from build123d import *

# Parameters (mm, degrees)
SKETCH1_R      = 5.9
EXTRUDE1_DEPTH = 10
FILLET1_R      = 2.8
EXTRUDE2_DEPTH = 8
FILLET2_R      = 0.2
EXTRUDE3_DEPTH = 9.8


with BuildPart() as part:
    # Sketch1 → Extrude1 (new body)
    with BuildSketch(Plane.XY):
        Circle(SKETCH1_R)
    extrude(amount=-EXTRUDE1_DEPTH)

    # Fillet1
    fillet1_edges = [part.edges().sort_by_distance(p)[0] for p in [
        (-5.9, 0, 0),
    ]]
    fillet(fillet1_edges, radius=FILLET1_R)

    # Sketch2 → Extrude2 (cut)
    with BuildSketch(Plane.XY):
        Polygon((-0.905, 2.315), (0.905, 2.315), (0.905, 0.905), (2.09345294, 0.905), (2.09345294, -0.905), (0.905, -0.905), (0.905, -2.273521567), (-0.905, -2.273521567), (-0.905, -0.905), (-2.345549018, -0.905), (-2.345549018, 0.905), (-0.905, 0.905), align=None)
    extrude(amount=-EXTRUDE2_DEPTH, mode=Mode.SUBTRACT)

    # Fillet2
    fillet2_edges = [part.edges().sort_by_distance(p)[0] for p in [
        (-0.905, 1.61, 0),
        (-1.625274509, 0.905, 0),
        (-2.345549018, 0, 0),
        (-1.625274509, -0.905, 0),
        (-0.905, -1.589260784, 0),
        (0, -2.273521567, 0),
        (0.905, -1.589260784, 0),
        (1.49922647, -0.905, 0),
        (2.09345294, 0, 0),
        (1.49922647, 0.905, 0),
        (0.905, 1.61, 0),
        (0, 2.315, 0),
    ]]
    fillet(fillet2_edges, radius=FILLET2_R)

    # Sketch3 → Extrude3 (add)
    with BuildSketch(Plane(origin=(0, 0, -10), x_dir=(-1, 0, 0), z_dir=(0, 0, -1))):
        with BuildLine():
            Line((-3.196218134, 0.9), (-8.1, 0.9))
            ThreePointArc((-8.1, 0.9), (-9, 0), (-8.1, -0.9))
            Line((-8.1, -0.9), (-3.196218134, -0.9))
            Line((-3.196218134, -0.9), (-3.196218134, 0.9))
        make_face()
        with BuildLine():
            Line((0.9, 3.376286761), (-0.9, 3.376286761))
            Line((-0.9, 3.376286761), (-0.9, 8.65))
            ThreePointArc((-0.9, 8.65), (0, 9.55), (0.9, 8.65))
            Line((0.9, 8.65), (0.9, 3.376286761))
        make_face()
        with BuildLine():
            Line((3.340273036, 0.9), (8.1, 0.9))
            ThreePointArc((8.1, 0.9), (9, 0), (8.1, -0.9))
            Line((8.1, -0.9), (3.340273036, -0.9))
            Line((3.340273036, -0.9), (3.340273036, 0.9))
        make_face()
        with BuildLine():
            Line((-0.9, -3.358279899), (0.9, -3.358279899))
            Line((0.9, -3.358279899), (0.9, -8.65))
            ThreePointArc((0.9, -8.65), (0, -9.55), (-0.9, -8.65))
            Line((-0.9, -8.65), (-0.9, -3.358279899))
        make_face()
    extrude(amount=-EXTRUDE3_DEPTH)

    # Sketch6 → Cut-Revolve3 (revolve, cut)
    with BuildSketch(Plane(origin=(0, 0, 0), x_dir=(0, 0, -1), z_dir=(1, 0, 0))):
        Polygon((2.318539135, -9.900453163), (-0.04993414, -9.900453163), (0.123609111, -4.036856485), align=None)
    revolve(axis=Axis((0, 0, -10.502496707), (0, 0, 1)), mode=Mode.SUBTRACT)


solid = part.part
CAD build for the part. Positions are in the model's coordinates, mm. A direction names the side the tool comes from. Coordinates: 2 decimals unless noted, no trailing zeros. Loops run counter-clockwise (first coordinate to the right, second up) from the corner with the lowest first, then second, coordinate; pieces in that order, holes last. Notation, with made-up numbers: (47, 81) -> (101, 81) arc R23 cw to (101, 91) -> close; hole circle Ø1 at (-35.75, 54.5). An arc over 180 degrees is marked (long way). One line per item, written item: value.
1. Slice it at B-B on x = 0. Write the cut outline in (y, z) (3 decimals).
Answers:
outline: (-9.55, -10) -> (9.55, -10) -> (9.55, -2.187) -> (4.241, -0.2) -> (4.139, -0.2) arc R2.8 ccw to (3.1, 0) -> (2.515, 0) arc R0.2 ccw to (2.315, -0.2) -> (2.315, -8) -> (-2.274, -8) -> (-2.274, -0.2) arc R0.2 ccw to (-2.474, 0) -> (-3.1, 0) arc R2.8 ccw to (-4.139, -0.2) -> (-4.241, -0.2) -> (-9.55, -2.187) -> close
2. Slice it at C-C on z = -1. Write the cut outline in (x, y) (3 decimals).
Answers:
outline: (-6.314, -0.9) -> (-5.167, -0.9) arc R5.245 ccw to (-0.9, -5.167) -> (-0.9, -6.314) arc R6.378 ccw to (0.9, -6.314) -> (0.9, -5.167) arc R5.245 ccw to (5.167, -0.9) -> (6.314, -0.9) arc R6.378 ccw to (6.314, 0.9) -> (5.167, 0.9) arc R5.245 ccw to (0.9, 5.167) -> (0.9, 6.314) arc R6.378 ccw to (-0.9, 6.314) -> (-0.9, 5.167) arc R5.245 ccw to (-5.167, 0.9) -> (-6.314, 0.9) arc R6.378 ccw to start; hole (-2.346, -0.905) -> (-0.905, -0.905) -> (-0.905, -2.274) -> (0.905, -2.274) -> (0.905, -0.905) -> (2.093, -0.905) -> (2.093, 0.905) -> (0.905, 0.905) -> (0.905, 2.315) -> (-0.905, 2.315) -> (-0.905, 0.905) -> (-2.346, 0.905) -> close
3. Which spindle directions (+Z, -Z, +X, -X, +Y, -Y) get a long thin tool onto all of the face, cutting with end or side? Do faces 1 (the face through (-2.346, 0, -4)), 2 (the face through (-0.02, -9.55, -5.99)). Say none if no direction does.
Answers:
face 1: +Z
face 2: +Z, -Z, -Y
4. Drill centre lines: line 1 (Y direction, x = 0.5, z = -5) (3 decimals); line 2 (Y direction, x = -7.5, z = -4.75); line 3 (Z direction, x = 0.5, y = -1.75). Where is each one in solid material? Low to high. Write a range as [from, to].
Answers:
line 1: y = [-9.398, -2.274], [2.315, 9.398]
line 2: y = [-0.9, 0.9]
line 3: z = [-10, -8]
5. Flat gauge pins, fed straight in: P1, Ø1.2, axis at x = -2, z = -3.5, coming from the -Y side; P2, Ø5, axis at y = 7.5, z = -6, coming from the -X side; P3, Ø6, axis at x = -4, z = -7.5, coming from the +Y side. Where does each tip first touch, or does it go through?
Answers:
P1: stops at y = -5.73
P2: stops at x = -3.13
P3: stops at y = 5.81
6. Slice it at A-A on z = -6.5. Write the cut outline in (x, y) (3 decimals), and give its area (3 significant figures).
Answers:
outline: (-8.1, -0.9) -> (-5.831, -0.9) arc R5.9 ccw to (-0.9, -5.831) -> (-0.9, -8.65) arc R0.9 ccw to (0.9, -8.65) -> (0.9, -5.831) arc R5.9 ccw to (5.831, -0.9) -> (8.1, -0.9) arc R0.9 ccw to (8.1, 0.9) -> (5.831, 0.9) arc R5.9 ccw to (0.9, 5.831) -> (0.9, 8.65) arc R0.9 ccw to (-0.9, 8.65) -> (-0.9, 5.831) arc R5.9 ccw to (-5.831, 0.9) -> (-8.1, 0.9) arc R0.9 ccw to start; hole (-2.346, -0.905) -> (-0.905, -0.905) -> (-0.905, -2.274) -> (0.905, -2.274) -> (0.905, -0.905) -> (2.093, -0.905) -> (2.093, 0.905) -> (0.905, 0.905) -> (0.905, 2.315) -> (-0.905, 2.315) -> (-0.905, 0.905) -> (-2.346, 0.905) -> close
area: 119 mm^2
7. Pull direction X, two halves, no side cores. Call faces 3 (the face through (9, 0, -6)), 4 (the face through (1.5, 0.905, -4)), 5 (the face through (2.093, 0, -4)), 6 (the face through (-0.9, -7, -5)): pulls with the +X half, pulls with the -X half, needs draft (parallel to the pull), parting line crosses it, or undercut.
Answers:
face 3: pulls with the +X half
face 4: undercut
face 5: undercut
face 6: pulls with the -X half
